Autodesk Fusion 360 part; units mm, degrees
sketch "bottom" plane through (0, 0, 0) normal (0, 0, 1) x (1, 0, 0)
  circle A0 centre (0, 0) radius 2.25
  circle A1 centre (0, 0) radius 5
  line L0 (5.04, 6.54) -> (-5.04, 6.54)
  line L1 (-6.54, 5.04) -> (-6.54, -5.04)
  line L2 (-5.04, -6.54) -> (5.04, -6.54)
  line L3 (6.54, -5.04) -> (6.54, 5.04)
  line L4 (6.54, 6.54) -> (-6.54, -6.54) construction
  line L5 (-6.54, 6.54) -> (6.54, -6.54) construction
  arc A2 (-5.04, 6.54) -> (-6.54, 5.04) centre (-5.04, 5.04) ccw
  arc A3 (6.54, 5.04) -> (5.04, 6.54) centre (5.04, 5.04) ccw
  arc A4 (5.04, -6.54) -> (6.54, -5.04) centre (5.04, -5.04) ccw
  arc A5 (-6.54, -5.04) -> (-5.04, -6.54) centre (-5.04, -5.04) ccw
  circle A6 centre (0, 0) radius 9.1
  circle A7 centre (0, 0) radius 11.25
  dimension "d1" = 4.5
  dimension "d2" = 10
  dimension "d3" = 13.08
  dimension "d4" = 13.08
  dimension "d5" = 1.5
  dimension "d6" = 18.2
  dimension "d7" = 22.5
extrude "Extrude1" add sketch "bottom" along normal blind 27.5 and the other way blind -7.5 contours L0 L1 L2 L3 A2 A3 A4 A5
extrude "Extrude2" add sketch "bottom" along normal blind 12.5 and the other way blind -7.5 contours A1
extrude "Extrude3" add sketch "bottom" along normal blind 12.5 contours A6
extrude "Extrude4" add sketch "bottom" along normal blind 2.5 contours A7
equation "d12 = 5.00 mm + 7.50 mm"
Source: CAD feature listing. Evaluate the final solid. Frame: model axes, mm. A direction names the side the tool comes from. Give positions to 0.01 mm unless a question says otherwise; leave off trailing zeros. Write each loop counter-clockwise with the first axis right and the second up, starting at its lowest first coordinate (ties: lowest second). Pieces come first, ordered by that corner, then holes.
1. Pull-direction query (Y, two-part tool) for faces 5 (the face through (5.19, 9.98, 1.23)), 6 (the face through (0, 6.54, 20)), 7 (the face through (-6.1, 6.1, 3.7)); classes: +Y half, -Y half, draft (parallel to the pull), parting line (faces both ways), or undercut.
2. Section query A-A (x = 0). Return the cut outline in (y, z), then the cut area to 3 significant figures.
3. Section query D-D (x = 8). Return the cut outline in (y, z), then the cut area to 3 significant figures.
4. First-contact query: pin 1 (1 mm diameter, centred on x = -8, y = 5.5, fed in from +Z); pin 2 (11 mm diameter, centred on x = 1.5, z = 20, fed in from +Y); pin 3 (2 mm diameter, centred on x = -6, z = 6, fed in from +Y). Flat tips, straight axial feed; report the tip coordinate or a pass-through.
5. Access query for faces 1 (the face through (0, -7, 12.5)), 2 (the face through (-6.1, 6.1, 19.9)), 3 (the face through (-6.54, 0, 4)), 4 (the face through (6.1, 6.1, 19.9)). Directions: +Z, -Z, +X, -X, +Y, -Y. A direction counts if a zero-diameter tool reaches every point of the face in a straight line with its end or side. Return the directions, or none.
6. Section query B-B (z = 2). Return the cut outline in (x, y), then the cut area to 3 significant figures.
7. Material intervals for line 1 along Y through (x, z) = (0, 9.05); line 2 along Y through (x, z) = (0, 23.5); line 3 along Z through (x, y) = (-4.5, 8.5), sorted ascending.
Output values:
1. face 5: parting line
1. face 6: +Y half
1. face 7: undercut
2. outline: (-11.25, 0) - (-6.54, 0) - (-6.54, 7.5) - (-2.25, 7.5) - (-2.25, 12.5) - (-5, 12.5) - (-5, 27.5) - (-6.54, 27.5) - (-6.54, 12.5) - (-9.1, 12.5) - (-9.1, 2.5) - (-11.25, 2.5) - close; (2.25, 7.5) - (6.54, 7.5) - (6.54, 0) - (11.25, 0) - (11.25, 2.5) - (9.1, 2.5) - (9.1, 12.5) - (6.54, 12.5) - (6.54, 27.5) - (5, 27.5) - (5, 12.5) - (2.25, 12.5) - close
2. area: 164 mm2
3. outline: (-7.91, 0) - (7.91, 0) - (7.91, 2.5) - (4.34, 2.5) - (4.34, 12.5) - (-4.34, 12.5) - (-4.34, 2.5) - (-7.91, 2.5) - close
3. area: 126 mm2
4. pin 1: stops at z = 2.5
4. pin 2: stops at y = 6.54
4. pin 3: stops at y = 7.6
5. face 1: +Z
5. face 2: +Z, -X, +Y
5. face 3: -Z
5. face 4: +Z, +X, +Y
6. outline: circle Ø22.5 at (0, 0); hole (-6.54, -5.04) arc R1.5 ccw to (-5.04, -6.54) - (5.04, -6.54) arc R1.5 ccw to (6.54, -5.04) - (6.54, 5.04) arc R1.5 ccw to (5.04, 6.54) - (-5.04, 6.54) arc R1.5 ccw to (-6.54, 5.04) - close
6. area: 228 mm2
7. line 1: y = -9.1 to -2.25, 2.25 to 9.1
7. line 2: y = -6.54 to -5, 5 to 6.54
7. line 3: z = 0 to 2.5
